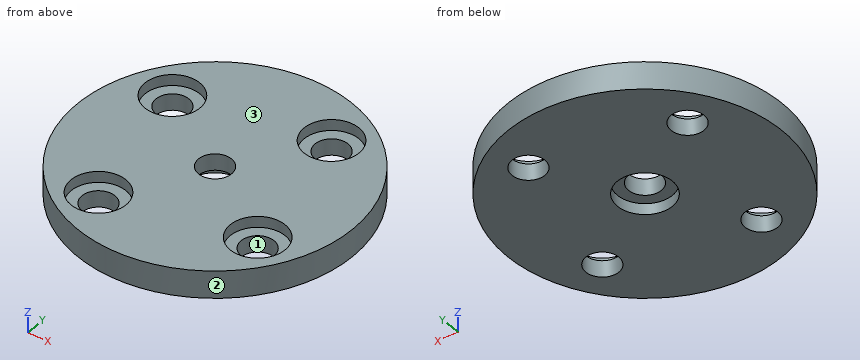
Autodesk Fusion 360 part; units mm, degrees
sketch "Sketch1" plane through (0, 0, 0) normal (0, 0, 1) x (1, 0, 0)
  circle A0 centre (0, 0) radius 25
  dimension "d1" = 50
extrude "Extrude1" add sketch "Sketch1" along normal blind 5
sketch "Sketch2" plane through (0, 0, 5) normal (0, 0, 1) x (-1, 0, 0)
  circle A0 centre (0, 0) radius 25
  circle A1 centre (15, -10) radius 3
  circle A2 centre (-10, -15) radius 3
  circle A3 centre (-15, 10) radius 3
  circle A4 centre (10, 15) radius 3
  dimension "d4" = 6
  dimension "d5" = 6
  dimension "d6" = 6
  dimension "d7" = 6
extrude "Extrude2" cut sketch "Sketch2" against normal blind 5 contours A1 | A2 | A3 | A4
sketch "Sketch3" plane through (0, 0, 5) normal (0, 0, 1) x (-1, 0, 0)
  circle A0 centre (-10, -15) radius 3
  circle A1 centre (-15, 10) radius 3
  circle A2 centre (15, -10) radius 3
  circle A3 centre (10, 15) radius 3
  circle A4 centre (0, 0) radius 25
  circle A5 centre (15, -10) radius 5
  circle A6 centre (-10, -15) radius 5
  circle A7 centre (-15, 10) radius 5
  circle A8 centre (10, 15) radius 5
  dimension "d10" = 10
  dimension "d11" = 10
  dimension "d12" = 10
  dimension "d13" = 10
extrude "Extrude3" cut sketch "Sketch3" against normal blind 2 contours A5 | A6 | A7 | A8
sketch "Sketch4" plane through (0, 0, 5) normal (0, 0, 1) x (-1, 0, 0)
  circle A0 centre (-10, -15) radius 5
  circle A1 centre (-15, 10) radius 5
  circle A2 centre (15, -10) radius 5
  circle A3 centre (10, 15) radius 5
  circle A4 centre (0, 0) radius 25
  circle A5 centre (0, 0) radius 3
  dimension "d16" = 6
extrude "Extrude4" cut sketch "Sketch4" against normal blind 21 contours A5
sketch "Sketch5" plane through (0, 0, 0) normal (0, 0, 1) x (1, 0, 0)
  circle A0 centre (0, 0) radius 5
  dimension "d19" = 10
extrude "Extrude5" cut sketch "Sketch5" along normal blind 2
Design review of the part built by this model. Coordinates are the model's own, in mm. Face numbers are marked on the shaded views. Give positions to 0.01 mm unless a question says otherwise; leave off trailing zeros. Loops run counter-clockwise (first coordinate to the right, second up) from the corner with the lowest first, then second, coordinate; pieces in that order, holes last. Notation, with made-up numbers: (-20, -18.75) -> (-10, -18.75) arc R19 cw to (-10, -1.75) -> close; hole circle Ø4 at (53.5, 53). An arc over 180 degrees is marked (long way). One line per question, with ' | ' between items. Start each with the question number.
(1) We need section C-C (z = 1.25). State the section outline as (x, y) points.
(2) Insertion check: P1, Ø1.5, axis at x = -19, z = 2, coming from the -Y side; P2, Ø1, axis at y = -10.5, z = 3.5, coming from the +X side; P3, Ø3, axis at x = 15.5, y = -8, coming from the +Z side; P4, Ø5.5, axis at x = 10, y = 15, coming from the -Z side. Each pin has a flat end and moves straight along its axis. Give the tip position at first contact, or say it passes through.
(3) We need section A-A (y = 0). State the section outline as (x, z) points, and give its area (3 significant figures).
(4) For line 1 (Y direction, x = -13, z = 4.15); line 2 (Y direction, x = 0, z = 1.3); line 3 (X direction, y = -13, z = 3.75), list the stretches that pass through material, from the lowest coordinate up.
(5) Draft analysis for pull direction X (two halves, no side actions). For the marked faces 1, 2 and 3, state which applies: +X half, -X half, draft (parallel to the pull), parting line (faces both ways), or undercut.
(6) We need section D-D (x = -21.5). State the section outline as (y, z) points.
The answers:
1) outline: circle Ø50 at (0, 0); hole circle Ø6 at (-15, 10); hole circle Ø6 at (-10, -15); hole circle Ø10 at (0, 0); hole circle Ø6 at (10, 15); hole circle Ø6 at (15, -10)
2) P1: stops at y = -17.09 | P2: stops at x = 22.91 | P3: stops at z = 3 | P4: passes through
3) outline: (-25, 0) -> (-5, 0) -> (-5, 2) -> (-3, 2) -> (-3, 5) -> (-25, 5) -> close; (3, 2) -> (5, 2) -> (5, 0) -> (25, 0) -> (25, 5) -> (3, 5) -> close | area: 212 mm^2
4) line 1: y = -21.35 to -19, -11 to 5.42, 14.58 to 21.35 | line 2: y = -25 to -5, 5 to 25 | line 3: x = -21.35 to -14.58, -5.42 to 11, 19 to 21.35
5) face 1: undercut | face 2: parting line | face 3: draft
6) outline: (-12.76, 0) -> (12.76, 0) -> (12.76, 5) -> (-12.76, 5) -> close
